Verification items for this drawing (mm, ordinates from the low corner). Coordinates: 2 decimals unless noted, no trailing zeros. Loops run counter-clockwise (first coordinate to the right, second up) from the corner with the lowest first, then second, coordinate; pieces in that order, holes last. Notation, with made-up numbers: (-39.5, 22) - (9.5, 22) arc R13 ccw to (9.5, 28) - close; hole circle Ø10 at (84, -31). An arc over 180 degrees is marked (long way). Write each question's results on one line, items separated by ' | '. Start each with the question number.
(1) Sectioned sample at A-A (y = 106.5). Enter the section's corners in (x, z).
(2) Sectioned sample at B-B (x = 57). Enter the section's corners in (y, z).
(3) Material ranges on probe 1 along X at (y, z) = (115.5, 99); probe 2 along Z at (x, y) = (148, 38); probe 3 along Y at (x, z) = (24, 103.5), recorded low to high.
(4) Go/stop test with flat-tipped pins: pin 1 Ø8 at (y, z) = (24.5, 70) entering from -X; pin 2 Ø3 at (x, z) = (83.5, 36) entering from -Y; pin 3 Ø1.5 at (y, z) = (69.5, 118) entering from -X. Record where each tip stops, or that it passes through.
(5) Sectioned sample at D-D (y = 60.5). Enter the section's corners in (x, z).
(6) Mould release check, pull along Z, two halves, no side actions. Record for the marked faces 1, 2 and 3: pulls with the +Z half, pulls with the -Z half, needs draft (parallel to the pull), parting line crosses it, or undercut.
(7) Sectioned sample at C-C (z = 57.5). Enter the section's corners in (x, y), plus the area to 3 significant figures.
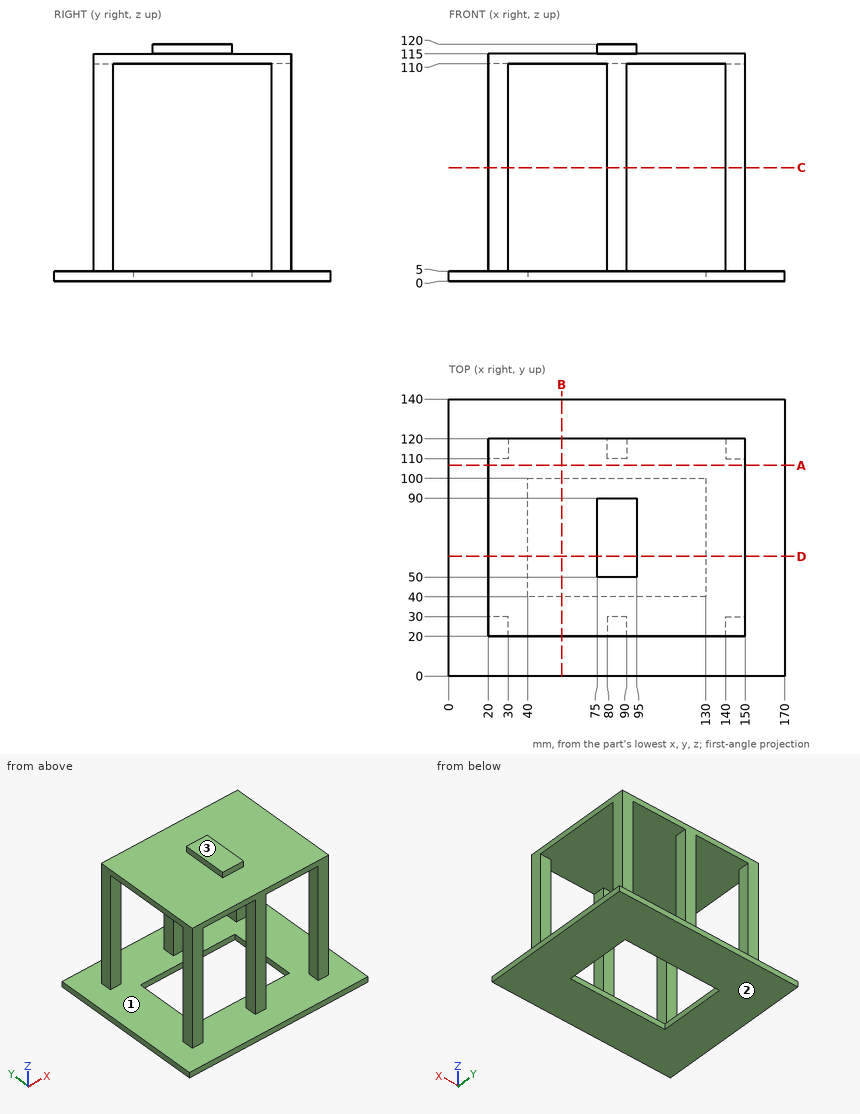
Outcome:
1) outline: (0, 0) - (170, 0) - (170, 5) - (0, 5) - close; (20, 110) - (150, 110) - (150, 115) - (20, 115) - close
2) outline: (0, 0) - (40, 0) - (40, 5) - (0, 5) - close; (20, 110) - (120, 110) - (120, 115) - (20, 115) - close; (100, 0) - (140, 0) - (140, 5) - (100, 5) - close
3) probe 1: x = 20 to 30, 80 to 90, 140 to 150 | probe 2: z = 0 to 5, 110 to 115 | probe 3: y = 20 to 30, 110 to 120
4) pin 1: stops at x = 20 | pin 2: stops at y = 20 | pin 3: stops at x = 75
5) outline: (0, 0) - (40, 0) - (40, 5) - (0, 5) - close; (20, 110) - (150, 110) - (150, 115) - (95, 115) - (95, 120) - (75, 120) - (75, 115) - (20, 115) - close; (130, 0) - (170, 0) - (170, 5) - (130, 5) - close
6) face 1: undercut | face 2: pulls with the -Z half | face 3: pulls with the +Z half
7) outline: (20, 20) - (30, 20) - (30, 30) - (20, 30) - close; (20, 110) - (30, 110) - (30, 120) - (20, 120) - close; (80, 20) - (90, 20) - (90, 30) - (80, 30) - close; (80, 110) - (90, 110) - (90, 120) - (80, 120) - close; (140, 20) - (150, 20) - (150, 30) - (140, 30) - close; (140, 110) - (150, 110) - (150, 120) - (140, 120) - close | area: 600 mm2
